from build123d import *

# Parameters (mm, degrees)
PAD_DEPTH       = 5
POCKET_DEPTH    = 5.001
POCKET001_DEPTH = 2.2


with BuildPart() as part:
    # Sketch → Pad (new body)
    with BuildSketch(Plane.XZ):
        Polygon((0, 0), (-13.102928, 36), (-46.742631, 36), (-46.742631, 46), (-6.742631, 46), (10, 0), align=None)
    extrude(amount=PAD_DEPTH)

    # Sketch001 (on Face8 of Pad) → Pocket (cut, through all)
    with BuildSketch(Plane.XZ.offset(5)):
        with BuildLine():
            ThreePointArc((-6.847488, 37.529023), (-9.029841, 38.546671), (-10.047488, 36.364318))
            Line((-10.047488, 36.364318), (1.843949, 3.692864))
            ThreePointArc((1.843949, 3.692864), (4.026301, 2.675216), (5.043949, 4.857568))
            Line((5.043949, 4.857568), (-6.847488, 37.529023))
        make_face()
    extrude(amount=-POCKET_DEPTH, mode=Mode.SUBTRACT)

    # Sketch002 (on Face5 of Pocket) → Pocket001 (cut)
    with BuildSketch(Plane.XZ.offset(5)):
        with BuildLine():
            Line((-40.742631, 45), (-23.942631, 43))
            ThreePointArc((-23.942631, 39), (-21.942631, 41), (-23.942631, 43))
            Line((-40.742631, 37), (-23.942631, 39))
            ThreePointArc((-40.742631, 45), (-44.742631, 41), (-40.742631, 37))
        make_face()
    extrude(amount=-POCKET001_DEPTH, mode=Mode.SUBTRACT)


solid = part.part
The listing builds one solid part. Answer for the finished solid, in the listing's coordinates (mm). A direction names the side the tool comes from. Give positions to 0.01 mm unless a question says otherwise; leave off trailing zeros. Loops run counter-clockwise (first coordinate to the right, second up) from the corner with the lowest first, then second, coordinate; pieces in that order, holes last.
Item 1: A cutting plane is placed at A-A (y = -1.45). Give the vertices of the cut face in (x, z), then the cut area to 3 significant figures.
Derived:
outline: (-46.74, 36) - (-13.1, 36) - (0, 0) - (10, 0) - (-6.74, 46) - (-46.74, 46) - close; hole (-10.05, 36.36) - (1.84, 3.69) arc R1.7 ccw to (5.04, 4.86) - (-6.85, 37.53) arc R1.7 ccw to start
area: 651 mm2
Item 2: A cutting plane is placed at D-D (z = 41). Give the vertices of the cut face in (x, y), then the cut area to 3 significant figures.
Derived:
outline: (-46.74, -5) - (-44.74, -5) - (-44.74, -2.8) - (-21.94, -2.8) - (-21.94, -5) - (-4.92, -5) - (-4.92, 0) - (-46.74, 0) - close
area: 159 mm2
Item 3: Find the intervals of material crossed by line 1 along Z through (x, y) = (-39, -2.7); line 2 along X through (y, z) = (-3.6, 42.5); line 3 along X through (y, z) = (-3.4, 3), in increasing order.
Derived:
line 1: z = 36 to 46
line 2: x = -46.74 to -44.45, -22.62 to -5.47
line 3: x = -1.09 to 2.32, 4.57 to 8.91
Item 4: A cutting plane is placed at B-B (z = 22). Give the vertices of the cut face in (x, y), then the cut area to 3 significant figures.
Derived:
outline: (-8.01, -5) - (-4.82, -5) - (-4.82, 0) - (-8.01, 0) - close; (-1.2, -5) - (1.99, -5) - (1.99, 0) - (-1.2, 0) - close
area: 31.9 mm2
Item 5: Each of these flat-tipped pins is pushed along its axis until it touches: pin 1 Ø1 at (y, z) = (-1.5, 10) entering from +X; pin 2 Ø9 at (x, z) = (-39, 41) entering from -Y; pin 3 Ø1.5 at (x, y) = (-36.5, -1.5) entering from -Z. Where does it stop, or does it pass through?
Derived:
pin 1: stops at x = 6.54
pin 2: stops at y = -5
pin 3: stops at z = 36
Item 6: A cutting plane is placed at C-C (x = -8). Give the vertices of the cut face in (y, z), then the cut area to 3 significant figures.
Derived:
outline: (-5, 21.98) - (0, 21.98) - (0, 30.74) - (-5, 30.74) - close; (-5, 38.59) - (0, 38.59) - (0, 46) - (-5, 46) - close
area: 80.8 mm2
Item 7: Determine the mould class of faces 1 (the flat face through (5, -2, 0)), 2 (the flat face through (-16, 0, 37)), 3 (the flat face through (-36, -2.8, 41)) for opening direction Z: +Z half, -Z half, draft (parallel to the pull), parting line (faces both ways), or undercut.
Derived:
face 1: -Z half
face 2: draft
face 3: undercut
Item 8: A tool of negligible diameter and unlimited length cuts with its end or side. For faces 4 (the cylindrical face through (-44.74, -3.92, 41.09)), 5 (the flat face through (-4.2, -2.5, 20.3)), 6 (the flat face through (-30, -2, 36)), from which of +Z, -Z, +X, -X, +Y, -Y can it reach the whole face along a straight path? Write none if from no direction.
Derived:
face 4: -Y
face 5: +Y, -Y
face 6: -Z, -X, +Y, -Y
